from build123d import *

# Parameters (mm, degrees)
SKETCH_1_R               = 6
SKETCH_1_R_2             = 2
EXTRUDE_1_DEPTH          = 9.25
SKETCH_2_R               = 6
SKETCH_2_R_2             = 2.5
EXTRUDE_2_DEPTH          = 9.25
CUT_EXTRUDE_1_DEPTH      = 10
CUT_EXTRUDE_1_DEPTH_BACK = 10


with BuildPart() as part:
    # 스케치1 → 보스-돌출1 (new body)
    with BuildSketch(Plane.XY):
        Circle(SKETCH_1_R)
        Circle(SKETCH_1_R_2, mode=Mode.SUBTRACT)
    extrude(amount=EXTRUDE_1_DEPTH)

    # 스케치2 → 보스-돌출2 (add)
    with BuildSketch(Plane.XY.offset(9.25)):
        Circle(SKETCH_2_R)
        Circle(SKETCH_2_R_2, mode=Mode.SUBTRACT)
    extrude(amount=EXTRUDE_2_DEPTH)

    # 스케치3 → 컷-돌출1 (cut, two sides: drawn at the far end of the back side and taken through both)
    with BuildSketch(Plane(origin=(0, 0, 0), x_dir=(1, 0, 0), z_dir=(0, 1, 0)).offset(-CUT_EXTRUDE_1_DEPTH_BACK)):
        with BuildLine():
            Line((-6, -2.5), (2, -2.5))
            ThreePointArc((2, -2.5), (2.25, -2.75), (2, -3))
            Line((2, -3), (-6, -3))
            Line((-6, -3), (-6, -2.5))
        make_face()
        with BuildLine():
            Line((-6, -12.5), (2, -12.5))
            ThreePointArc((2, -12.5), (2.25, -12.75), (2, -13))
            Line((2, -13), (-6, -13))
            Line((-6, -13), (-6, -12.5))
        make_face()
        with BuildLine():
            Line((6, -6), (-2, -6))
            ThreePointArc((-2, -6), (-2.25, -5.75), (-2, -5.5))
            Line((-2, -5.5), (6, -5.5))
            Line((6, -5.5), (6, -6))
        make_face()
        with BuildLine():
            Line((6, -16), (-2, -16))
            ThreePointArc((-2, -16), (-2.25, -15.75), (-2, -15.5))
            Line((-2, -15.5), (6, -15.5))
            Line((6, -15.5), (6, -16))
        make_face()
    extrude(amount=CUT_EXTRUDE_1_DEPTH + CUT_EXTRUDE_1_DEPTH_BACK, mode=Mode.SUBTRACT)


solid = part.part
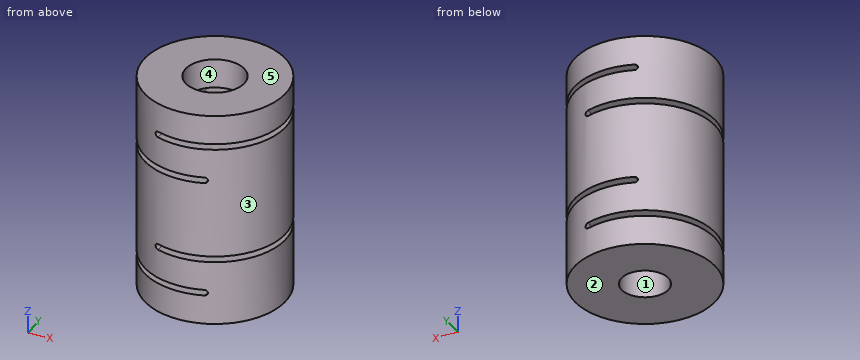
Geometry check sheet. Reference: the model listing, model coordinates, mm. Face numbers are marked on the shaded views. A direction names the side the tool comes from. Round coordinates to 2 decimals unless told otherwise and drop trailing zeros. Order: outer loops, then holes, each group sorted by start corner. A loop starts at its lowest first (then second) coordinate and runs counter-clockwise, first axis right, second up. Notation, with made-up numbers: M 65.5,-11 L 113.5,-11 A26 ccw 113.5,17 Z; hole C 24,5.25 d2. An arc over 180 degrees is marked long. Answer in a Markdown table with one row per item.
(1) Sectioned sample at C-C, the plane x = 5. Record the cut outline in (y, z).
Responses:
| item | result |
|---|---|
| outline | M -3.32,0 L 3.32,0 L 3.32,5.5 L -3.32,5.5 Z; M -3.32,6 L 3.32,6 L 3.32,15.5 L -3.32,15.5 Z; M -3.32,16 L 3.32,16 L 3.32,18.5 L -3.32,18.5 Z |
(2) Sectioned sample at B-B, the plane z = 11.5. Record the cut outline in (x, y), and give its area (3 significant figures).
Responses:
| item | result |
|---|---|
| outline | C 0,0 d12; hole C 0,0 d5 |
| area | 93.5 mm² |
(3) Tool access check on the marked faces 4 and 5. Record the directions out of +Z, -Z, +X, -X, +Y, -Y that give a thin tool (end or side, any length) a straight path to the whole face; none if there is none.
Responses:
| item | result |
|---|---|
| face 4 | +Z |
| face 5 | +Z, +X, -X, +Y, -Y |
(4) Scan lines: probe 1 along Z at (x, y) = (-4.75, 0.5); probe 2 along Z at (x, y) = (-2, -3); probe 3 along Z at (x, y) = (4.5, -1). Record each from-to range of solid material in increasing order. Write a range as from..to.
Responses:
| item | result |
|---|---|
| probe 1 | z = 0..2.5, 3..12.5, 13..18.5 |
| probe 2 | z = 0..2.5, 3..5.5, 6..12.5, 13..15.5, 16..18.5 |
| probe 3 | z = 0..5.5, 6..15.5, 16..18.5 |
(5) Sectioned sample at A-A, the plane x = 0. State how many separate pieces and enclosed holes the cut face has, and give its area (3 significant figures).
Responses:
| item | result |
|---|---|
| separate pieces | 10 |
| enclosed holes | 0 |
| area | 124 mm² |
(6) Draft check along Y on the marked faces 1, 2 and 3. Enter one of: released by +Y, released by -Y, zero draft, split by the parting line, or undercut.
Responses:
| item | result |
|---|---|
| face 1 | undercut |
| face 2 | zero draft |
| face 3 | split by the parting line |
(7) Sectioned sample at D-D, the plane y = 4.5. Record the cut outline in (x, z).
Responses:
| item | result |
|---|---|
| outline | M -3.97,0 L 3.97,0 L 3.97,5.5 L -2,5.5 A0.25 cw -2,6 L 3.97,6 L 3.97,15.5 L -2,15.5 A0.25 cw -2,16 L 3.97,16 L 3.97,18.5 L -3.97,18.5 L -3.97,13 L 2,13 A0.25 cw 2,12.5 L -3.97,12.5 L -3.97,3 L 2,3 A0.25 cw 2,2.5 L -3.97,2.5 Z |
(8) Go/stop test with flat-tipped pins: P1, Ø2.5, axis at x = -0.5, y = 1, coming from the -Z side; P2, Ø1, axis at x = -2.5, z = 13, coming from the +Y side; P3, Ø1.5, axis at x = 1, y = 1, coming from the +Z side; P4, Ø1, axis at y = -3.5, z = 16.5, coming from the +X side. Record where each tip stops, or that it passes through.
Responses:
| item | result |
|---|---|
| P1 | stops at z = 0 |
| P2 | stops at y = 5.66 |
| P3 | stops at z = 9.25 |
| P4 | stops at x = 5.2 |
